CAD build for the part. Positions are in the model's coordinates, mm. Face numbers are marked on the shaded views. A direction names the side the tool comes from. Round coordinates to 2 decimals unless told otherwise and drop trailing zeros. Loops run counter-clockwise (first coordinate to the right, second up) from the corner with the lowest first, then second, coordinate; pieces in that order, holes last. Notation, with made-up numbers: (-27, 30.25) - (25, 30.25) arc R26 cw to (25, 55.25) - close; hole circle Ø8 at (26, 65.5). An arc over 180 degrees is marked (long way). One line per question, with ' | ' between items.
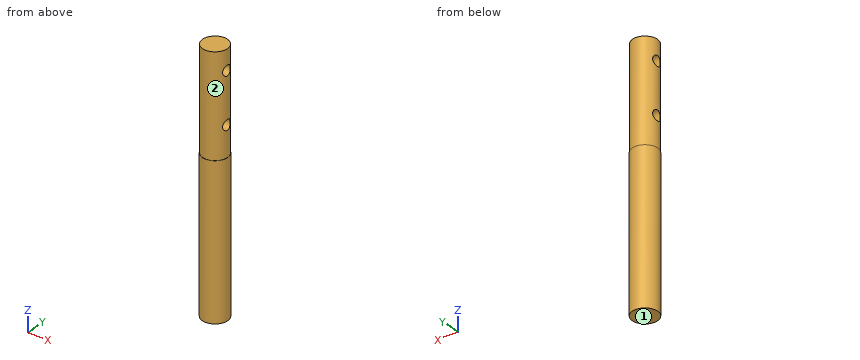
```python
from build123d import *

# Parameters (mm, degrees)
SKETCH1_R               = 25
BOSS_EXTRUDE1_DEPTH     = 250
CUT_EXTRUDE1_DEPTH      = 253.487623459
CUT_EXTRUDE1_DEPTH_BACK = 253.487623459
SKETCH2_R               = 10.05
SKETCH3_OUTSIDE_W       = 152.996
SKETCH3_OUTSIDE_H       = 152.996
SKETCH3_OUTSIDE_R       = 24.61
CUT_EXTRUDE2_DEPTH      = 200


with BuildPart() as part:
    # Sketch1 → Boss-Extrude1 (new, symmetric)
    with BuildSketch(Plane.XY):
        Circle(SKETCH1_R)
    extrude(amount=BOSS_EXTRUDE1_DEPTH, both=True)

    # Sketch2 → Cut-Extrude1 (cut, two sides: drawn at the far end of the back side and taken through both)
    with BuildSketch(Plane(origin=(0, 0, 0), x_dir=(0, 0, -1), z_dir=(1, 0, 0)).offset(-CUT_EXTRUDE1_DEPTH_BACK)):
        with Locations(Location((-210, 0, 0), (0, 0, 180))):
            Circle(SKETCH2_R)
        with Locations(Location((-110, 0, 0), (0, 0, 180))):
            Circle(SKETCH2_R)
    extrude(amount=CUT_EXTRUDE1_DEPTH + CUT_EXTRUDE1_DEPTH_BACK, mode=Mode.SUBTRACT)

    # Sketch3 outside → Cut-Extrude2 (cut)
    with BuildSketch(Plane.XY.offset(250)):
        Rectangle(SKETCH3_OUTSIDE_W, SKETCH3_OUTSIDE_H)
        Circle(SKETCH3_OUTSIDE_R, mode=Mode.SUBTRACT)
    extrude(amount=-CUT_EXTRUDE2_DEPTH, mode=Mode.SUBTRACT)


solid = part.part
```
(1) Probe L1, parallel to Z at x = 21.5, y = -1; L2, parallel to Y at x = -2, z = 110; L3, parallel to Z at x = -11.5, y = -8. List the from-to ranges inside material, lowest first.
Results found:
L1: z = -250 to 100, 120 to 200, 220 to 250 | L2: y = -24.53 to -10.05, 10.05 to 24.53 | L3: z = -250 to 103.92, 116.08 to 203.92, 216.08 to 250
(2) Cut at B-B, the plane x = -6. Write the cut outline in (y, z).
Results found:
outline: (-24.27, -250) - (24.27, -250) - (24.27, 50) - (23.87, 50) - (23.87, 250) - (-23.87, 250) - (-23.87, 50) - (-24.27, 50) - close; hole circle Ø20.1 at (0, 110); hole circle Ø20.1 at (0, 210)
(3) Cut at D-D, the plane y = -20. Write the cut outline in (x, z).
Results found:
outline: (-15, -250) - (15, -250) - (15, 50) - (14.34, 50) - (14.34, 250) - (-14.34, 250) - (-14.34, 50) - (-15, 50) - close
(4) Cut at C-C, the plane z = -110. Write the cut outline in (x, y), then the cut area to 3 significant figures.
Results found:
outline: circle Ø50 at (0, 0) | area: 1,960 mm²
(5) Tool access for the marked faces 1 and 2: list every direction of +Z, -Z, +X, -X, +Y, -Y with a clear straight run to the whole face (end or side of a thin tool).
Results found:
face 1: -Z, +X, -X, +Y, -Y | face 2: +Z
(6) Cut at A-A, the plane y = 0. Write the cut outline in (x, z), then the cut area to 3 significant figures.
Results found:
outline: (-25, -250) - (25, -250) - (25, 50) - (24.61, 50) - (24.61, 99.95) - (-24.61, 99.95) - (-24.61, 50) - (-25, 50) - close; (-24.61, 120.05) - (24.61, 120.05) - (24.61, 199.95) - (-24.61, 199.95) - close; (-24.61, 220.05) - (24.61, 220.05) - (24.61, 250) - (-24.61, 250) - close | area: 22,900 mm²
(7) Drop flat-ended pins along their axis: P1, Ø12, axis at y = 16, z = -23, coming from the +X side; P2, Ø23, axis at y = 0, z = 210, coming from the -X side; P3, Ø1.5, axis at y = -1, z = 29.5, coming from the -X side. Give the stop position or say it passes through.
Results found:
P1: stops at x = 22.91 | P2: stops at x = -24.61 | P3: stops at x = -25
